```python
from build123d import *

# Parameters (mm, degrees)
F0_W     = 50
F0_H     = 50
F0_W_2   = 40
F0_H_2   = 40
F1_DEPTH = 35
F2_W     = 50
F2_H     = 50
F3_DEPTH = 25
F4_SIZE  = 24.99999


# Not quite as in the source:
# - a fillet or chamfer is up to 0.001 mm smaller than in the source, because OpenCascade refuses the exact size


with BuildPart() as f1:
    # F0 (on Front) → F1 (new body)
    with BuildSketch(Plane.XZ):
        with Locations((25, 25)):
            Rectangle(F0_W, F0_H)
        with Locations((25, 25)):
            Rectangle(F0_W_2, F0_H_2, mode=Mode.SUBTRACT)
    extrude(amount=-F1_DEPTH)

    # F2 (on face) → F3 (join)
    with BuildSketch(Plane(origin=(0, 35, 0), x_dir=(-1, 0, 0), z_dir=(0, 1, 0))):
        with Locations((-25, 25)):
            Rectangle(F2_W, F2_H)
    extrude(amount=F3_DEPTH)

    # F4 (size 25 in the source; OpenCascade refuses exactly that, so slightly less here)
    f4_edges = [f1.edges().sort_by_distance(p)[0] for p in [
        (0, 60, 25),
        (50, 60, 25),
    ]]
    chamfer(f4_edges, length=F4_SIZE)


solid = f1.part
```
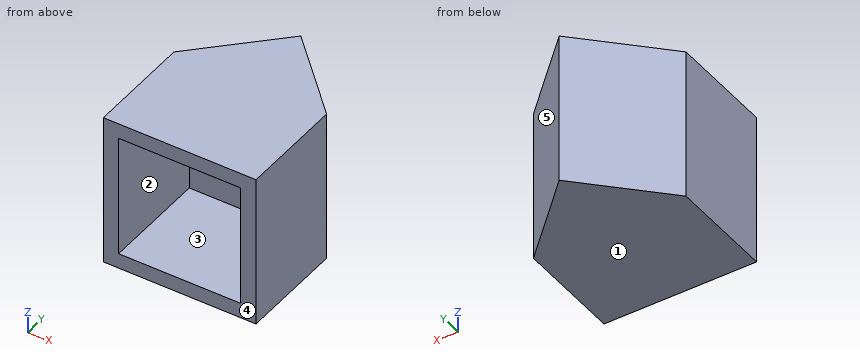
Can you work these out from the model? Positions are in its coordinate system, mm. Face numbers are marked on the shaded views. A direction names the side the tool comes from. Coordinates: 2 decimals unless noted, no trailing zeros. Write each loop counter-clockwise with the first axis right and the second up, starting at its lowest first coordinate (ties: lowest second). Pieces come first, ordered by that corner, then holes. Notation, with made-up numbers: M -10,15.25 L 42,15.25 A29 ccw 42,45.25 Z; hole C 85.25,47 d6. An arc over 180 degrees is marked long. Answer as CSV lines item,"result".
Item 1: I'm going to push flat-ended pins straight in: P1, Ø8, axis at y = 47, z = 36.5, coming from the +X side; P2, Ø2, axis at x = 43.5, z = 26.5, coming from the -Y side. Where does each tip first touch, or does it pass through?
Geometry results:
P1,"stops at x = 42"
P2,"stops at y = 35"
Item 2: Imagine slicing it at C-C on x = 20. List the corners of the cut face in (y, z) for me.
Geometry results:
outline,"M 0,0 L 55,0 L 55,50 L 0,50 L 0,45 L 35,45 L 35,5 L 0,5 Z"
Item 3: Imagine slicing it at A-A on y = 22. List the corners of the cut face in (x, z) for me.
Geometry results:
outline,"M 0,0 L 50,0 L 50,50 L 0,50 Z; hole M 5,5 L 45,5 L 45,45 L 5,45 Z"
Item 4: On a 3-axis mill with a long thin cutter (end or side, diameter ignored), from which of +Z, -Z, +X, -X, +Y, -Y can I reach the whole of each face in a straight line? I mean the marked faces 1 and 2. Say none if no direction works.
Geometry results:
face 1,"-Z, +X, -X, +Y, -Y"
face 2,"-Y"
Item 5: We'd pull the mould along X, two halves only. Please class the marked faces 3, 4 and 5: +X half, -X half, draft (parallel to the pull), parting line (faces both ways), or undercut.
Geometry results:
face 3,"undercut"
face 4,"draft"
face 5,"+X half"
Item 6: Please list where these lines run through material, in increasing order: line 1 along Z through (x, y) = (6, 22); line 2 along X through (y, z) = (40, 25).
Geometry results:
line 1,"z = 0 to 5, 45 to 50"
line 2,"x = 5 to 45"
Item 7: Imagine slicing it at D-D on y = 37. List the corners of the cut face in (x, z) for me, plus the area to 3 significant figures.
Geometry results:
outline,"M 2,0 L 48,0 L 48,50 L 2,50 Z"
area,"2,300 mm2"
